The figure shows three views and two pictorial views of one solid part (mm, origin at its lowest corner). Answer the questions. A direction names the side the tool comes from. Give positions to 0.01 mm unless a question says otherwise; leave off trailing zeros. Order: outer loops, then holes, each group sorted by start corner. A loop starts at its lowest first (then second) coordinate and runs counter-clockwise, first axis right, second up. Notation, with made-up numbers: (-29, 64) - (-23, 64) arc R14 cw to (-23, 77) - close; hole circle Ø11 at (83, 25). An arc over 180 degrees is marked (long way). Use a Markdown table: item, result. Add a question column.
1. A cutting plane is placed at D-D on y = 12. Determine the outline of the cut face in (x, z), and give its area (3 significant figures).
2. A cutting plane is placed at A-A on z = 12.5. Determine the outline of the cut face in (x, y), and give its area (4 significant figures).
3. For a pull along Z with two mould halves and no side action, classify the marked faces 1, 2 and 3 as released by +Z, released by -Z, zero draft, split by the parting line, or undercut.
4. Flat-ended cylindrical pins translate along their axes: P1, Ø5, axis at x = 12.5, y = 18, coming from the +Z side; P2, Ø5, axis at x = 11.5, y = 9.5, coming from the -Z side; P3, Ø5, axis at x = 14.5, y = 19, coming from the -Z side. Find the tip coordinate at first contact, or state that the pin passes through.
5. Which of the six approach directions +Z, -Z, +X, -X, +Y, -Y give full straight-line access (tool end or side, diameter ignored) to the marked faces 4, 5 and 6?
6. A cutting plane is placed at C-C on y = 18. Determine the outline of the cut face in (x, z), and give its area (3 significant figures).
7. A cutting plane is placed at B-B on x = 12.5. State how many separate pieces and enclosed holes the cut face has, and give its area (4 significant figures).
8. Consider L1, parallel to Y at x = 12.5, z = 17.15; L2, parallel to Y at x = 16.5, z = 21.25; L3, parallel to Y at x = 12.5, z = 4. Determine where each line is inside the solid, lowest interval first.
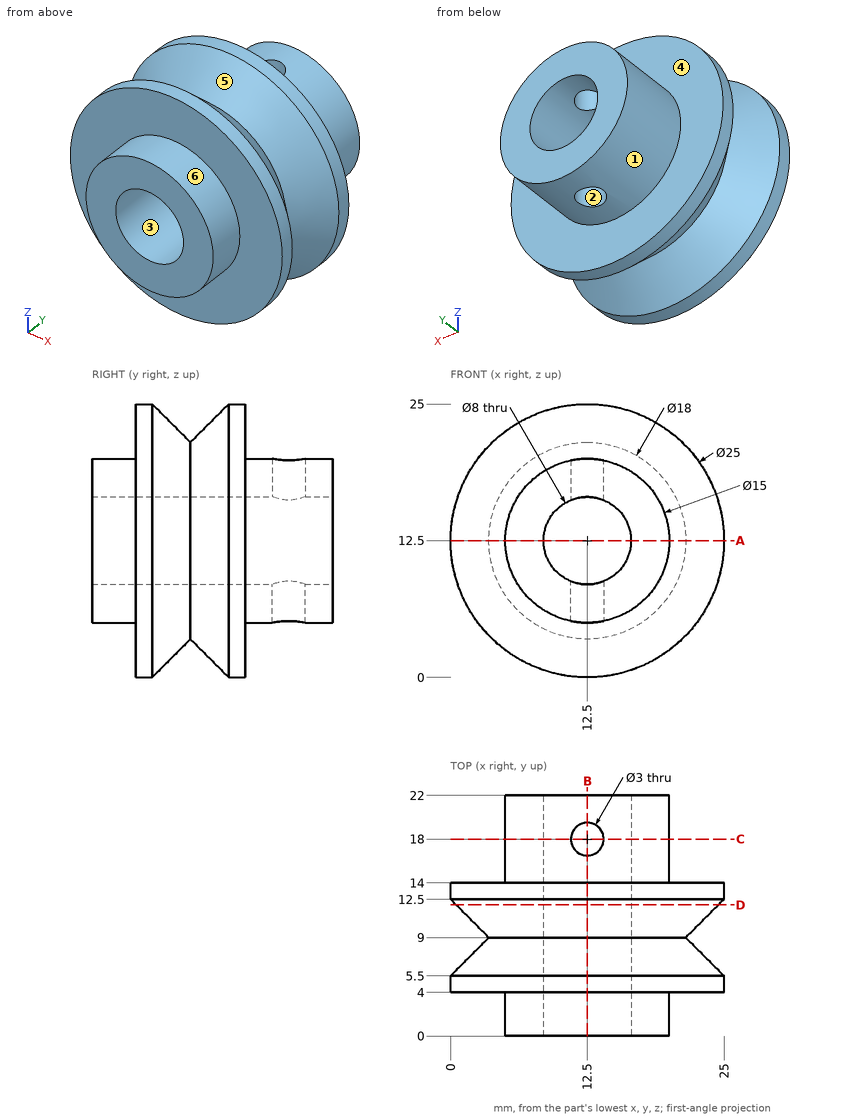
Output values:
| question | item | result |
|---|---|---|
| 1 | outline | circle Ø24 at (12.5, 12.5); hole circle Ø8 at (12.5, 12.5) |
| 1 | area | 402 mm² |
| 2 | outline | (0, 4) - (5, 4) - (5, 0) - (8.5, 0) - (8.5, 22) - (5, 22) - (5, 14) - (0, 14) - (0, 12.5) - (3.5, 9) - (0, 5.5) - close; (16.5, 0) - (20, 0) - (20, 4) - (25, 4) - (25, 5.5) - (21.5, 9) - (25, 12.5) - (25, 14) - (20, 14) - (20, 22) - (16.5, 22) - close |
| 2 | area | 229.5 mm² |
| 3 | face 1 | split by the parting line |
| 3 | face 2 | zero draft |
| 3 | face 3 | undercut |
| 4 | P1 | z = 20 |
| 4 | P2 | z = 0.53 |
| 4 | P3 | z = 5 |
| 5 | face 4 | +Y |
| 5 | face 5 | none |
| 5 | face 6 | -Y |
| 6 | outline | (11, 5.15) - (11, 8.79) arc R4 cw to (11, 16.21) - (11, 19.85) arc R7.5 ccw to start; (14, 5.15) arc R7.5 ccw to (14, 19.85) - (14, 16.21) arc R4 cw to (14, 8.79) - close |
| 6 | area | 105 mm² |
| 7 | separate pieces | 4 |
| 7 | enclosed holes | 0 |
| 7 | area | 208.5 mm² |
| 8 | L1 | 0 to 16.5, 19.5 to 22 |
| 8 | L2 | 4 to 8.38, 9.62 to 14 |
| 8 | L3 | 4 to 14 |
